Design review of the part built by this model. Coordinates are the model's own, in mm. Face numbers are marked on the shaded views. A direction names the side the tool comes from. Coordinates: 2 decimals unless noted, no trailing zeros. Loops run counter-clockwise (first coordinate to the right, second up) from the corner with the lowest first, then second, coordinate; pieces in that order, holes last. Notation, with made-up numbers: (82, 41) -> (94, 41) arc R29 cw to (94, 77) -> close; hole circle Ø7 at (20.5, -39). An arc over 180 degrees is marked (long way). Answer in a Markdown table with one row per item.
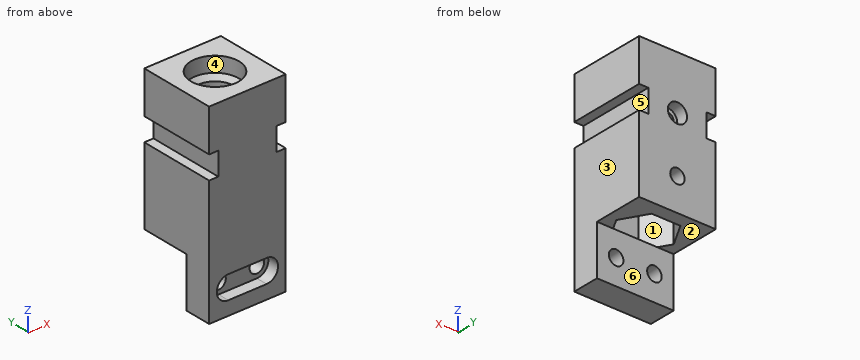
Autodesk Inventor part; units mm, degrees
ref_plane "YZ Plane" through (0, 0, 0) normal (1, 0, 0) x (0, 1, 0)
ref_plane "XZ Plane" through (0, 0, 0) normal (0, 1, 0) x (-1, 0, 0)
ref_plane "XY Plane" through (0, 0, 0) normal (0, 0, 1) x (1, 0, 0)
sketch "Boceto1" plane through (0, 0, 0) normal (0, 1, 0) x (-1, 0, 0)
  line L0 (0, 0) -> (50.8, 0)
  line L1 (50.8, -93.98) -> (0, -93.98)
  line L2 (50.8, -27.94) -> (44.704, -27.94)
  line L3 (44.704, -27.94) -> (44.704, -43.18)
  line L4 (44.704, -43.18) -> (50.8, -43.18)
  line L5 (6.096, -27.94) -> (0, -27.94)
  line L6 (0, -43.18) -> (6.096, -43.18)
  line L7 (6.096, -43.18) -> (6.096, -27.94)
  line L8 (50.8, 0) -> (50.8, -27.94)
  line L9 (50.8, -43.18) -> (50.8, -93.98)
  line L10 (0, -93.98) -> (0, -43.18)
  line L11 (0, -27.94) -> (0, 0)
  dimension "d0" = 50.8
  dimension "d1" = 93.98
  dimension "d2" = 27.94
  dimension "d3" = 15.24
  dimension "d5" = 27.94
  dimension "d6" = 15.24
extrude "BaseAlta" add sketch "Boceto1" along normal blind 50.8
sketch "Boceto2" plane through (0, 0, 0) normal (0, 1, 0) x (-1, 0, 0)
  line L0 (0, -93.98) -> (50.8, -93.98)
  line L1 (0, -93.98) -> (50.8, -93.98)
  line L2 (50.8, -93.98) -> (50.8, -127)
  line L3 (50.8, -127) -> (0, -127)
  line L4 (0, -127) -> (0, -93.98)
  point P0 (0, 0)
  dimension "d10" = 50.8
  dimension "d11" = 33.02
extrude "BaseBaja" add sketch "Boceto2" along normal blind 17.78
sketch "Boceto4" plane through (0, 50.8, -93.98) normal (0, 0, -1) x (-1, 0, 0)
  circle A0 centre (25.4, -25.4) radius 19.05 construction
  line L0 (0, -50.8) -> (50.8, -50.8) construction
  line L1 (0, -33.02) -> (0, 0) construction
  line L2 (6.35, -25.4) -> (15.875, -8.9022)
  line L3 (15.875, -8.9022) -> (34.925, -8.9022)
  line L4 (34.925, -8.9022) -> (44.45, -25.4)
  line L5 (44.45, -25.4) -> (34.925, -41.8978)
  line L6 (34.925, -41.8978) -> (15.875, -41.8978)
  line L7 (15.875, -41.8978) -> (6.35, -25.4)
  dimension "d19" = 38.1
  dimension "d20" = 25.4
  dimension "d21" = 25.4
extrude "Hexagono" cut sketch "Boceto4" against normal blind 43.18
sketch "Boceto6" plane through (0, 17.78, 0) normal (0, 1, 0) x (1, 0, 0)
  circle A0 centre (-38.1, 110.236) radius 4.826
  circle A1 centre (-12.7, 110.236) radius 4.826
  line L0 (0, 127) -> (-50.8, 127)
  line L1 (-50.8, 127) -> (-50.8, 93.98)
  line L2 (0, 93.98) -> (0, 127)
  point P0 (0, 0)
  dimension "d35" = 9.652
  dimension "d36" = 9.652
  dimension "d37" = 16.764
  dimension "d38" = 16.764
  dimension "d39" = 12.7
  dimension "d40" = 12.7
  dimension "d41" = 25.4
extrude "DosAgujeros" cut sketch "Boceto6" against normal blind 10.16
sketch "Boceto7" plane through (0, 0, 0) normal (0, -1, 0) x (1, 0, 0)
  circle A0 centre (-12.7, -110.236) radius 4.826 construction
  circle A1 centre (-38.1, -110.236) radius 4.826 construction
  arc A2 (-12.7, -117.856) -> (-12.7, -102.616) centre (-12.7, -110.236) ccw
  arc A3 (-38.1, -102.616) -> (-38.1, -117.856) centre (-38.1, -110.236) ccw
  line L0 (-12.7, -117.856) -> (-38.1, -117.856)
  line L1 (-12.7, -102.616) -> (-38.1, -102.616)
  line L2 (0, -43.18) -> (0, -127)
  line L3 (0, -127) -> (-50.8, -127)
  line L4 (-50.8, -127) -> (-50.8, -43.18)
  point P0 (0, 0)
  dimension "d44" = 15.24
  dimension "d45" = 15.24
  dimension "d46" = 12.7
  dimension "d47" = 16.764
  dimension "d48" = 12.7
  dimension "d49" = 16.764
extrude "AgujeroInferior" cut sketch "Boceto7" against normal blind 7.62
sketch "Boceto8" plane through (-50.8, 0, 0) normal (0, 0, 1) x (1, 0, 0)
  line L0 (0, 0) -> (50.8, 0)
  line L1 (0, 0) -> (0, 50.8)
  point P0 (25.4, 25.4)
  dimension "d52" = 25.4
  dimension "d53" = 25.4
hole "Agujero" at (-25.4, 25.4, 0) direction (0, 0, -1) diameter 25.4 depth 50.8 tip angle 118 counterbore diameter 31.75 counterbore depth 13.208
sketch "Boceto9" plane through (0, 50.8, 0) normal (0, 1, 0) x (1, 0, 0)
  circle A0 centre (-25.4, 72.39) radius 4.7625
  line L0 (-50.8, 93.98) -> (-50.8, 43.18)
  line L1 (0, 93.98) -> (-50.8, 93.98)
  point P0 (0, 0)
  dimension "d61" = 9.525
  dimension "d62" = 25.4
  dimension "d63" = 21.59
extrude "HoyoSuperior" cut sketch "Boceto9" against normal blind 12.7
sketch "Boceto10" plane through (0, 50.8, 0) normal (0, 1, 0) x (1, 0, 0)
  line L0 (-50.8, 27.94) -> (-50.8, 0)
  line L1 (-50.8, 0) -> (0, 0)
  point P0 (-25.4, 35.56)
  dimension "d66" = 25.4
  dimension "d67" = 35.56
hole "Agujero3" at (-25.4, 50.8, -35.56) direction (0, -1, 0) diameter 7.874 depth 12.7 counterbore diameter 12.7 counterbore depth 7.62
chamfer "Chaflán1" distance 3.175 angle 45 1 edges at (-25.4, 41.275, -13.208) measured on face at (-24.1336, 10.7371, -13.208)
equation "\"d38\" = d37"
properties part number "Box A01209499"
(1) For pin 1 (4.5 mm diameter, centred on y = 37, z = -35.5, fed in from +X); pin 2 (10 mm diameter, centred on x = -25.4, z = -35.56, fed in from +Y); pin 3 (11 mm diameter, centred on x = -38.1, z = -110.236, fed in from -Y), all flat-tipped, find the tip position at first contact; note any pin that passes through.
Evaluation:
| item | result |
|---|---|
| pin 1 | stops at x = -6.1 |
| pin 2 | stops at y = 43.18 |
| pin 3 | stops at y = 7.62 |
(2) Tool access review of the marked faces 4, 5 and 6: name each direction out of +Z, -Z, +X, -X, +Y, -Y from which nothing blocks a thin tool from reaching the whole face with its end or side.
Evaluation:
| item | result |
|---|---|
| face 4 | +Z |
| face 5 | +X, +Y, -Y |
| face 6 | -Z, +X, -X, +Y |
(3) Take a section at B-B on z = -35.56. Give the boundary of the cut face in (x, y), and give its area (3 significant figures).
Evaluation:
| item | result |
|---|---|
| outline | (-44.7, 0) -> (-6.1, 0) -> (-6.1, 50.8) -> (-19.05, 50.8) -> (-19.05, 43.18) -> (-21.46, 43.18) -> (-21.46, 38.1) -> (-29.34, 38.1) -> (-29.34, 43.18) -> (-31.75, 43.18) -> (-31.75, 50.8) -> (-44.7, 50.8) -> close; hole circle Ø25.4 at (-25.4, 25.4) |
| area | 1,320 mm² |
(4) To check wall thickness, follow probe 1 along Z at (x, y) = (-38, 15); probe 2 along Z at (x, y) = (-2, 38); probe 3 along Z at (x, y) = (-38.1, 12). State the ranges of each line that lie inside material, in increasing order.
Evaluation:
| item | result |
|---|---|
| probe 1 | z = -127 to -115.06, -105.41 to -93.98, -50.8 to 0 |
| probe 2 | z = -93.98 to -43.18, -27.94 to 0 |
| probe 3 | z = -127 to -115.06, -105.41 to 0 |
(5) Take a section at C-C on y = 14.5. Count the separate pieces of the cut face and the enclosed holes in it, and give its area (3 significant figures).
Evaluation:
| item | result |
|---|---|
| separate pieces | 1 |
| enclosed holes | 2 |
| area | 4,240 mm² |
(6) Draft analysis for pull direction Z (two halves, no side actions). For the marked faces 1, 2 and 3, state which applies: pulls with the +Z half, pulls with the -Z half, needs draft (parallel to the pull), parting line crosses it, or undercut.
Evaluation:
| item | result |
|---|---|
| face 1 | undercut |
| face 2 | pulls with the -Z half |
| face 3 | needs draft |
(7) Take a section at A-A on y = 5. Give the boundary of the cut face in (x, z).
Evaluation:
| item | result |
|---|---|
| outline | (-50.8, -127) -> (0, -127) -> (0, -43.18) -> (-6.1, -43.18) -> (-6.1, -27.94) -> (0, -27.94) -> (0, 0) -> (-50.8, 0) -> (-50.8, -27.94) -> (-44.7, -27.94) -> (-44.7, -43.18) -> (-50.8, -43.18) -> close; hole (-38.1, -117.86) -> (-12.7, -117.86) arc R7.62 ccw to (-12.7, -102.62) -> (-38.1, -102.62) arc R7.62 ccw to start |
